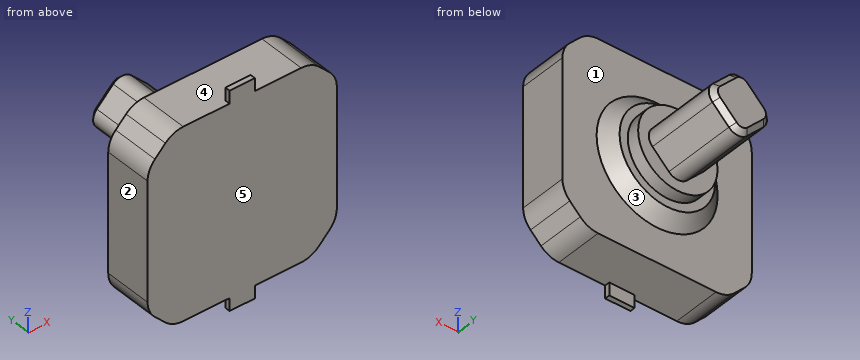
from build123d import *

# Parameters (mm, degrees)
BOSS_EXTRUDE1_DEPTH = 1.9
BOSS_EXTRUDE2_DEPTH = 6
SKETCH3_R           = 2.397073563
BOSS_EXTRUDE3_DEPTH = 0.5
BOSS_EXTRUDE3_TAPER = 45
SKETCH4_R           = 1.57169904
BOSS_EXTRUDE4_DEPTH = 0.5
SKETCH5_W           = 1
SKETCH5_H           = 0.5
BOSS_EXTRUDE5_DEPTH = 0.2
CHAMFER1_SIZE       = 0.2


with BuildPart() as part:
    # Sketch1 → Boss-Extrude1 (new body)
    with BuildSketch(Plane(origin=(0, 0, 0), x_dir=(1, 0, 0), z_dir=(0, 1, 0))):
        with BuildLine():
            Line((-3.457106781, 3.042893219), (-3.042893219, 3.457106781))
            ThreePointArc((-3.042893219, 3.457106781), (-2.71846987, 3.673879533), (-2.335786438, 3.75))
            Line((-2.335786438, 3.75), (2.335786438, 3.75))
            ThreePointArc((2.335786438, 3.75), (2.71846987, 3.673879533), (3.042893219, 3.457106781))
            Line((3.042893219, 3.457106781), (3.457106781, 3.042893219))
            ThreePointArc((3.457106781, 3.042893219), (3.673879533, 2.71846987), (3.75, 2.335786438))
            Line((3.75, 2.335786438), (3.75, -2.335786438))
            ThreePointArc((3.75, -2.335786438), (3.673879533, -2.71846987), (3.457106781, -3.042893219))
            Line((3.457106781, -3.042893219), (3.042893219, -3.457106781))
            ThreePointArc((3.042893219, -3.457106781), (2.71846987, -3.673879533), (2.335786438, -3.75))
            Line((2.335786438, -3.75), (-2.335786438, -3.75))
            ThreePointArc((-2.335786438, -3.75), (-2.71846987, -3.673879533), (-3.042893219, -3.457106781))
            Line((-3.042893219, -3.457106781), (-3.457106781, -3.042893219))
            ThreePointArc((-3.457106781, -3.042893219), (-3.673879533, -2.71846987), (-3.75, -2.335786438))
            Line((-3.75, -2.335786438), (-3.75, 2.335786438))
            ThreePointArc((-3.75, 2.335786438), (-3.673879533, 2.71846987), (-3.457106781, 3.042893219))
        make_face()
    extrude(amount=BOSS_EXTRUDE1_DEPTH)

    # Sketch2 → Boss-Extrude2 (add)
    with BuildSketch(Plane(origin=(0, 0, 0), x_dir=(1, 0, 0), z_dir=(0, 1, 0))):
        with BuildLine():
            Line((0.353553391, -1.004091629), (1.004091629, -0.353553391))
            ThreePointArc((1.004091629, -0.353553391), (1.150538239, 0), (1.004091629, 0.353553391))
            Line((1.004091629, 0.353553391), (0.353553391, 1.004091629))
            ThreePointArc((0.353553391, 1.004091629), (0, 1.150538239), (-0.353553391, 1.004091629))
            Line((-0.353553391, 1.004091629), (-1.004091629, 0.353553391))
            ThreePointArc((-1.004091629, 0.353553391), (-1.150538239, 0), (-1.004091629, -0.353553391))
            Line((-1.004091629, -0.353553391), (-0.353553391, -1.004091629))
            ThreePointArc((-0.353553391, -1.004091629), (0, -1.150538239), (0.353553391, -1.004091629))
        make_face()
    extrude(amount=BOSS_EXTRUDE2_DEPTH)

    # Sketch3 → Boss-Extrude3 (add)
    with BuildSketch(Plane(origin=(0, 1.9, 0), x_dir=(1, 0, 0), z_dir=(0, 1, 0))):
        Circle(SKETCH3_R)
    extrude(amount=BOSS_EXTRUDE3_DEPTH, taper=BOSS_EXTRUDE3_TAPER)

    # Sketch4 → Boss-Extrude4 (add)
    with BuildSketch(Plane(origin=(0, 2.4, 0), x_dir=(1, 0, 0), z_dir=(0, 1, 0))):
        Circle(SKETCH4_R)
    extrude(amount=BOSS_EXTRUDE4_DEPTH)

    # Sketch5 → Boss-Extrude5 (add)
    with BuildSketch(Plane(origin=(0, 0, 0), x_dir=(1, 0, 0), z_dir=(0, 1, 0))):
        with Locations((0, -4)):
            Rectangle(SKETCH5_W, SKETCH5_H)
        with Locations((0, 4)):
            Rectangle(SKETCH5_W, SKETCH5_H)
    extrude(amount=BOSS_EXTRUDE5_DEPTH)

    # Chamfer1
    chamfer1_edges = [part.edges().sort_by_distance(p)[0] for p in [
        (0, 6, 1.150538239),
        (0.67882251, 6, 0.67882251),
        (1.150538239, 6, 0),
        (0.67882251, 6, -0.67882251),
        (0, 6, -1.150538239),
        (-0.67882251, 6, -0.67882251),
        (-1.150538239, 6, 0),
        (-0.67882251, 6, 0.67882251),
    ]]
    chamfer(chamfer1_edges, length=CHAMFER1_SIZE)


solid = part.part
Verification items for the finished model (mm, model axes). Face numbers are marked on the shaded views. A direction names the side the tool comes from. Coordinates: 2 decimals unless noted, no trailing zeros. Order: outer loops, then holes, each group sorted by start corner. A loop starts at its lowest first (then second) coordinate and runs counter-clockwise, first axis right, second up.
1. Sectioned sample at B-B, the plane y = 4. Record the cut outline in (x, z), and give its area (3 significant figures).
Results found:
outline: (-1, -0.35) - (-0.35, -1) arc R0.5 ccw to (0.35, -1) - (1, -0.35) arc R0.5 ccw to (1, 0.35) - (0.35, 1) arc R0.5 ccw to (-0.35, 1) - (-1, 0.35) arc R0.5 ccw to start
area: 3.47 mm2
2. Release check for a two-part mould opening along Y. For the marked faces 3, 4 and 5 record: +Y half, -Y half, draft (parallel to the pull), parting line (faces both ways), or undercut.
Results found:
face 3: +Y half
face 4: draft
face 5: -Y half
3. Go/stop test with flat-tipped pins: pin 1 Ø1.5 at (y, z) = (2.5, 0.5) entering from -X; pin 2 Ø2 at (y, z) = (3.5, -0.5) entering from -X; pin 3 Ø0.6 at (x, y) = (0.5, 1) entering from -Z. Record where each tip stops, or that it passes through.
Results found:
pin 1: stops at x = -3.75
pin 2: stops at x = -1.57
pin 3: stops at z = -3.75
4. Set-up check for the marked faces 1 and 2: record each of +Z, -Z, +X, -X, +Y, -Y from which the full face is reachable in a straight line by a thin tool's end or side.
Results found:
face 1: +Y
face 2: +Z, -Z, -X, +Y, -Y
5. Scan lines: line 1 (Y direction, x = -2.5, z = 1.75); line 2 (Z direction, x = -1.75, y = 1.75); line 3 (Y direction, x = 1.5, z = 0.75). Record each from-to range of solid material in increasing order.
Results found:
line 1: y = 0 to 1.9
line 2: z = -3.75 to 3.75
line 3: y = 0 to 2.4
6. Sectioned sample at A-A, the plane x = 0. Record the cut outline in (y, z).
Results found:
outline: (0, -4.25) - (0.2, -4.25) - (0.2, -3.75) - (1.9, -3.75) - (1.9, -2.4) - (2.4, -1.9) - (2.4, -1.57) - (2.9, -1.57) - (2.9, -1.15) - (5.8, -1.15) - (6, -0.95) - (6, 0.95) - (5.8, 1.15) - (2.9, 1.15) - (2.9, 1.57) - (2.4, 1.57) - (2.4, 1.9) - (1.9, 2.4) - (1.9, 3.75) - (0.2, 3.75) - (0.2, 4.25) - (0, 4.25) - close
7. Sectioned sample at C-C, the plane x = 2.75. Record the cut outline in (y, z).
Results found:
outline: (0, -3.66) - (1.9, -3.66) - (1.9, 3.66) - (0, 3.66) - close
